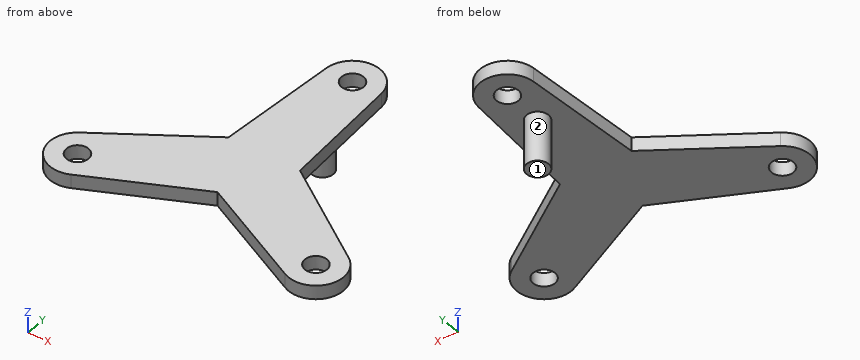
```python
from build123d import *

# Parameters (mm, degrees)
BOSS_EXTRUDE1_DEPTH = 5
SKETCH3_R           = 4
CUT_EXTRUDE1_DEPTH  = 5
SKETCH4_R           = 4
PEG_DEPTH           = 18


with BuildPart() as part:
    # Sketch1 → Boss-Extrude1 (new body)
    with BuildSketch(Plane.XY):
        with BuildLine():
            Line((-38.916331436, -83.987341772), (0, -65))
            Line((0, -65), (38.916331436, -83.987341772))
            ThreePointArc((38.916331436, -83.987341772), (51.961524227, -80), (48.8920671, -66.708860759))
            Line((48.8920671, -66.708860759), (12.990381057, -42.5))
            Line((12.990381057, -42.5), (9.975735664, 0.696202532))
            ThreePointArc((9.975735664, 0.696202532), (0, 10), (-9.975735664, 0.696202532))
            Line((-9.975735664, 0.696202532), (-12.990381057, -42.5))
            Line((-12.990381057, -42.5), (-48.8920671, -66.708860759))
            ThreePointArc((-48.8920671, -66.708860759), (-51.961524227, -80), (-38.916331436, -83.987341772))
        make_face()
    extrude(amount=BOSS_EXTRUDE1_DEPTH)

    # Sketch3 → Cut-Extrude1 (cut)
    with BuildSketch(Plane(origin=(0, 0, 0), x_dir=(-1, 0, 0), z_dir=(0, 0, -1))):
        with Locations((0, 30)):
            Circle(SKETCH3_R)
        Circle(SKETCH3_R)
        with Locations((-43.301270189, -75)):
            Circle(SKETCH3_R)
        with Locations((43.301270189, -75)):
            Circle(SKETCH3_R)
    extrude(amount=-CUT_EXTRUDE1_DEPTH, mode=Mode.SUBTRACT)

    # Sketch4 → peg (add)
    with BuildSketch(Plane(origin=(0, 0, 0), x_dir=(-1, 0, 0), z_dir=(0, 0, -1))):
        with Locations((0, -14.5)):
            Circle(SKETCH4_R)
    extrude(amount=PEG_DEPTH)


solid = part.part
```
Can you work these out from the model? Positions are in its coordinate system, mm. Face numbers are marked on the shaded views. A direction names the side the tool comes from. Give positions to 0.01 mm unless a question says otherwise; leave off trailing zeros. Write each loop counter-clockwise with the first axis right and the second up, starting at its lowest first coordinate (ties: lowest second). Pieces come first, ordered by that corner, then holes. Notation, with made-up numbers: (-13, 5.25) - (10, 5.25) arc R14 ccw to (10, 30.25) - close; hole circle Ø4 at (85.25, 5). An arc over 180 degrees is marked (long way). Write item = value, one per line. Start each with the question number.
1. Imagine slicing it at D-D (y = -75). Please give me the cut outline in (x, z).
2. Imagine slicing it at B-B (x = -40.5). Please give me the cut outline in (y, z).
3. Imagine slicing it at C-C (y = -14.5). Please give me the cut outline in (x, z).
4. On a 3-axis mill with a long thin cutter (end or side, diameter ignored), from which of +Z, -Z, +X, -X, +Y, -Y can I reach the whole of each face in a straight line? I mean the marked faces 1 and 2. Say none if no direction works.
5. For pin 1 (8 mm diameter, centred on y = -11, z = -6.5, fed in from +X); pin 2 (1.5 mm diameter, centred on y = -37.5, z = 0, fed in from -X); pin 3 (10 mm diameter, centred on x = 29.5, y = -62.5, fed in from -Z), each with a flat end and sliding along its axis, tell me the tip position at first contact or that it passes through.
6. Please list where these lines run through material, in increasing order: line 1 (Y direction, x = 0, z = 2.3); line 2 (Z direction, x = 38, y = -64.5); line 3 (Y direction, x = -3, z = 3).
7. Imagine slicing it at A-A (z = 3.75). Please give me the cut outline in (x, y).
Worked answers:
q1.outline = (-53.3, 0) - (-47.3, 0) - (-47.3, 5) - (-53.3, 5) - close; (-39.3, 0) - (-20.5, 0) - (-20.5, 5) - (-39.3, 5) - close; (20.5, 0) - (39.3, 0) - (39.3, 5) - (20.5, 5) - close; (47.3, 0) - (53.3, 0) - (53.3, 5) - (47.3, 5) - close
q2.outline = (-84.6, 0) - (-77.86, 0) - (-77.86, 5) - (-84.6, 5) - close; (-72.14, 0) - (-61.05, 0) - (-61.05, 5) - (-72.14, 5) - close
q3.outline = (-11.04, 0) - (-4, 0) - (-4, -18) - (4, -18) - (4, 0) - (11.04, 0) - (11.04, 5) - (-11.04, 5) - close
q4.face_1 = -Z, +X, -X, +Y, -Y
q4.face_2 = -Z
q5.pin_1 = 4
q5.pin_2 = -12.69
q5.pin_3 = 0
q6.line_1 = -65 to -4, 4 to 10
q6.line_2 = 0 to 5
q6.line_3 = -66.46 to -2.65, 2.65 to 9.54
q7.outline = (-48.89, -66.71) arc R10 ccw to (-38.92, -83.99) - (0, -65) - (38.92, -83.99) arc R10 ccw to (48.89, -66.71) - (12.99, -42.5) - (9.98, 0.7) arc R10 ccw to (-9.98, 0.7) - (-12.99, -42.5) - close; hole circle Ø8 at (-43.3, -75); hole circle Ø8 at (0, 0); hole circle Ø8 at (43.3, -75)
